Source: three-view drawing plus pictorial views. Frame: mm from the lowest corner of the part. Coordinates: 2 decimals unless noted, no trailing zeros. Write each loop counter-clockwise with the first axis right and the second up, starting at its lowest first coordinate (ties: lowest second). Pieces come first, ordered by that corner, then holes. Notation, with made-up numbers: (81, 59) -> (87, 59) arc R22 cw to (87, 88) -> close; hole circle Ø5 at (9.5, 8.5). An arc over 180 degrees is marked (long way). One line per question, with ' | ' between items. Start each with the question number.
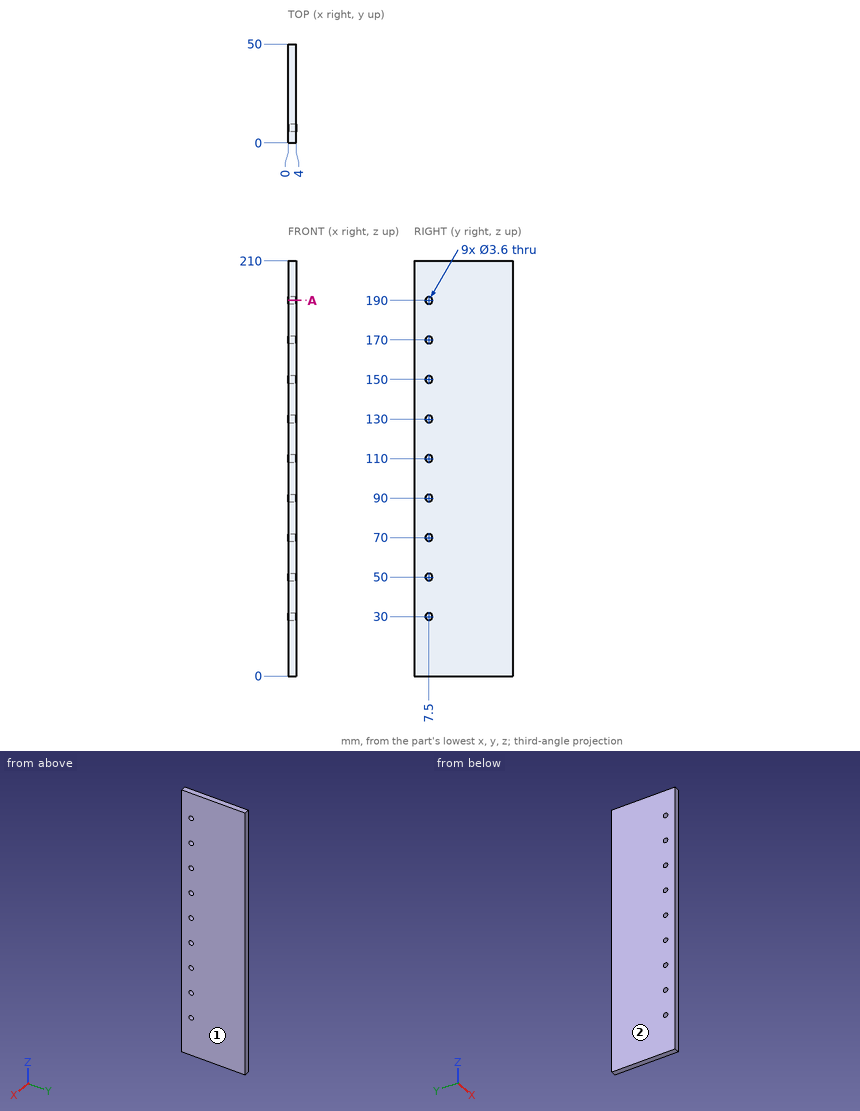
1) Pull-direction query (X, two-part tool) for the marked faces 1 and 2; classes: released by +X, released by -X, zero draft, split by the parting line, or undercut.
2) Section A-A, the plane z = 190. Return loops of the section in (x, y).
3) Ray query, line 1 (Y direction, x = 1.2, z = 50); line 2 (Y direction, x = 0.55, z = 30.5). Return the intervals inside material, ascending.
Answer block:
1) face 1: released by +X | face 2: released by -X
2) outline: (0, 0) -> (4, 0) -> (4, 5.7) -> (0, 5.7) -> close; (0, 9.3) -> (4, 9.3) -> (4, 50) -> (0, 50) -> close
3) line 1: y = 0 to 5.7, 9.3 to 50 | line 2: y = 0 to 5.77, 9.23 to 50
